Geometry: final body of the model. Coordinates: model frame, mm. Give positions to 0.01 mm unless a question says otherwise; leave off trailing zeros. Loops run counter-clockwise (first coordinate to the right, second up) from the corner with the lowest first, then second, coordinate; pieces in that order, holes last. Notation, with made-up numbers: (71, 86.25) -> (101, 86.25) arc R27 cw to (101, 121.25) -> close; hole circle Ø11 at (-19, -29). An arc over 180 degrees is marked (long way). Answer in a Markdown table with one row per item. Add a question column.
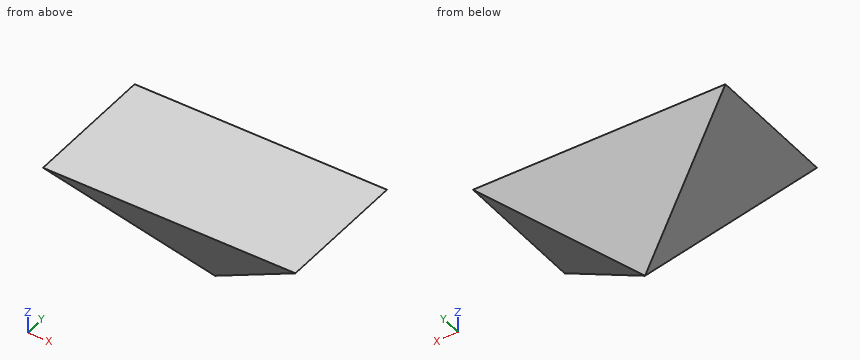
from build123d import *

# Parameters (mm, degrees)
BOSS_EXTRUDE1_DEPTH = 90.101349
CUT_EXTRUDE3_DEPTH  = 257.717103907
CUT_EXTRUDE4_DEPTH  = 202.563222837


with BuildPart() as part:
    # 3DSketch1 → Boss-Extrude1 (new body)
    with BuildSketch(Plane(origin=(-103.731361149, 50.299698024, -48.298204463), x_dir=(0.8813808665660824, -0.4724063590291962, 0), z_dir=(0, 0, 1))):
        Polygon((0, 0), (182.853673959, 98.006709275), (235.383737233, 0), (52.530063274, -98.006709275), align=None)
    extrude(amount=-BOSS_EXTRUDE1_DEPTH)

    # Sketch3 → Cut-Extrude3 (cut, through all)
    with BuildSketch(Plane.ZY.offset(103.731361149)):
        Polygon((-48.298204463, 50.299698024), (-132.298204463, -5.298689116), (-48.298204463, -60.897076257), (-138.399553935, -60.897076257), (-138.399553935, 50.299698024), align=None)
    extrude(amount=-CUT_EXTRUDE3_DEPTH, mode=Mode.SUBTRACT)

    # Sketch2 → Cut-Extrude4 (cut, through all)
    with BuildSketch(Plane(origin=(0, 50.299698024, 0), x_dir=(1, 0, 0), z_dir=(0, 1, 0))):
        Polygon((-103.731361149, 48.298204463), (0, 132.298204463), (103.731361149, 48.298204463), (103.731361149, 138.399553935), (-103.731361149, 138.399553935), align=None)
    extrude(amount=-CUT_EXTRUDE4_DEPTH, mode=Mode.SUBTRACT)


solid = part.part
(1) Pin query (flat end, axial travel): pin 1 Ø5 at (y, z) = (3.5, -95.5) entering from -X; pin 2 Ø6 at (y, z) = (30.5, -58.5) entering from +X; pin 3 Ø3 at (y, z) = (19, -81.5) entering from +X. Return the tip coordinate at first contact, or that it passes through.
(2) Cut plane A-A on x = -49. Return the cut outline in (y, z).
(3) Cut plane B-B on z = -106. Return the cut outline in (x, y).
(4) Material intervals for line 1 along X through (y, z) = (-26, -88.5); line 2 along Z through (x, y) = (-67, 6.5); line 3 along Z through (x, y) = (-3.5, 32.5), sorted ascending. Write a range as from..to.
Answer list:
| question | item | result |
|---|---|---|
| 1 | pin 1 | stops at x = -48.53 |
| 1 | pin 2 | stops at x = 94.84 |
| 1 | pin 3 | stops at x = 64.58 |
| 2 | outline | (-60.9, -48.3) -> (-31.56, -92.62) -> (20.96, -92.62) -> (50.3, -48.3) -> close |
| 3 | outline | (-32.48, -22.71) -> (32.48, -22.71) -> (32.48, 12.11) -> (-32.48, 12.11) -> close |
| 4 | line 1 | x = -54.09..54.09 |
| 4 | line 2 | z = -78.04..-48.3 |
| 4 | line 3 | z = -75.19..-48.3 |
